Here's how the part is built. I have some questions about the finished solid (model axes, mm). Coordinates: 2 decimals unless noted, no trailing zeros. Write each loop counter-clockwise with the first axis right and the second up, starting at its lowest first coordinate (ties: lowest second). Pieces come first, ordered by that corner, then holes. Notation, with made-up numbers: (30.5, 76) -> (35.5, 76) arc R25 ccw to (35.5, 99) -> close; hole circle Ø6 at (37.25, 5.25). An arc over 180 degrees is marked (long way). Answer in a Markdown table with one row per item. Add a question column.
from build123d import *

# Parameters (mm, degrees)
BOSS_EXTRUDE1_DEPTH = 133.35
SKETCH2_R           = 21
CUT_EXTRUDE1_DEPTH  = 187.593999065
SKETCH3_W           = 133.35
SKETCH3_H           = 3.175
BOSS_EXTRUDE2_DEPTH = 3.175
FILLET1_R           = 3.175
SKETCH5_R           = 15
CUT_EXTRUDE2_DEPTH  = 189.467318942
SKETCH6_R           = 6.0325
CUT_EXTRUDE3_DEPTH  = 189.467318942
SKETCH7_R           = 3.175
CUT_EXTRUDE4_DEPTH  = 189.472240296
SKETCH15_R          = 2.5
CUT_EXTRUDE8_DEPTH  = 189.467318942
SKETCH18_R          = 30.1625
SKETCH18_R_2        = 21
BOSS_EXTRUDE3_DEPTH = 2.688354466


with BuildPart() as part:
    # Sketch1 → Boss-Extrude1 (new body)
    with BuildSketch(Plane.XY):
        Polygon((110.49, -69.425000088), (0, 0), (0, 3.175), (110.49, -66.250000088), align=None)
    extrude(amount=BOSS_EXTRUDE1_DEPTH)

    # Sketch2 → Cut-Extrude1 (cut, through all)
    with BuildSketch(Plane(origin=(1.430283892, 2.276299128, 0), x_dir=(0.8467258159330607, -0.5320295035357462, 0), z_dir=(0.5320295035357462, 0.8467258159330607, 0))):
        with Locations(Location((42.760806326, -41.91, 0), (0, 0, 180))):
            Circle(SKETCH2_R)
    extrude(amount=-CUT_EXTRUDE1_DEPTH, mode=Mode.SUBTRACT)

    # Sketch3 → Boss-Extrude2 (add)
    with BuildSketch(Plane(origin=(110.49, 0, 0), x_dir=(0, 0, -1), z_dir=(1, 0, 0))):
        with Locations((-66.675, -67.837500088)):
            Rectangle(SKETCH3_W, SKETCH3_H)
    extrude(amount=BOSS_EXTRUDE2_DEPTH)

    # Fillet1
    fillet1_edges = [part.edges().sort_by_distance(p)[0] for p in [
        (113.665, -66.250000088, 66.675),
    ]]
    fillet(fillet1_edges, radius=FILLET1_R - 0.0001)  # a hair under: the kernel refuses the full size

    # Sketch5 → Cut-Extrude2 (cut, through all)
    with BuildSketch(Plane(origin=(1.430283892, 2.276299128, 0), x_dir=(0.8467258159330606, -0.5320295035357464, 0), z_dir=(0.5320295035357464, 0.8467258159330606, 0))):
        with Locations(Location((17.360806326, -101.6, 0), (0, 0, 180))):
            Circle(SKETCH5_R)
        with Locations(Location((58.000806326, -101.6, 0), (0, 0, 180))):
            Circle(SKETCH5_R)
    extrude(amount=-CUT_EXTRUDE2_DEPTH, mode=Mode.SUBTRACT)

    # Sketch6 → Cut-Extrude3 (cut, through all)
    with BuildSketch(Plane(origin=(1.430283892, 2.276299128, 0), x_dir=(0.8467258159330606, -0.5320295035357464, 0), z_dir=(0.5320295035357464, 0.8467258159330606, 0))):
        with Locations(Location((90.701690059, -66.675, 0), (0, 0, 180))):
            Circle(SKETCH6_R)
        with Locations(Location((90.701690059, -47.625, 0), (0, 0, 180))):
            Circle(SKETCH6_R)
        with Locations(Location((90.701690059, -28.575, 0), (0, 0, 180))):
            Circle(SKETCH6_R)
        with Locations(Location((90.701690059, -85.725, 0), (0, 0, 180))):
            Circle(SKETCH6_R)
        with Locations(Location((90.701690059, -104.775, 0), (0, 0, 180))):
            Circle(SKETCH6_R)
    extrude(amount=-CUT_EXTRUDE3_DEPTH, mode=Mode.SUBTRACT)

    # Sketch7 → Cut-Extrude4 (cut, through all)
    with BuildSketch(Plane(origin=(0, 0, 0), x_dir=(0.8467258159330607, -0.5320295035357464, 0), z_dir=(-0.5320295035357463, -0.8467258159330606, 0))):
        with Locations((105.090883732, 123.825)):
            Circle(SKETCH7_R)
        with Locations((25.4, 123.825)):
            Circle(SKETCH7_R)
        with Locations((25.4, 9.525)):
            Circle(SKETCH7_R)
        with Locations((105.090883732, 9.525)):
            Circle(SKETCH7_R)
    extrude(amount=-CUT_EXTRUDE4_DEPTH, mode=Mode.SUBTRACT)

    # Sketch15 → Cut-Extrude8 (cut, through all)
    with BuildSketch(Plane(origin=(1.430283892, 2.276299128, 0), x_dir=(0.8467258159330606, -0.5320295035357464, 0), z_dir=(0.5320295035357464, 0.8467258159330606, 0))):
        with Locations(Location((17.360806326, -76.2, 0), (0, 0, 180))):
            Circle(SKETCH15_R)
        with Locations(Location((76.731690059, -66.675, 0), (0, 0, 180))):
            Circle(SKETCH15_R)
        with Locations(Location((58.000806326, -76.2, 0), (0, 0, 180))):
            Circle(SKETCH15_R)
    extrude(amount=-CUT_EXTRUDE8_DEPTH, mode=Mode.SUBTRACT)

    # Sketch18 → Boss-Extrude3 (add)
    with BuildSketch(Plane(origin=(1.430283892, 2.276299128, 0), x_dir=(0.8467258159330606, -0.5320295035357464, 0), z_dir=(0.5320295035357464, 0.8467258159330606, 0))):
        with Locations((42.760806326, -41.91)):
            Circle(SKETCH18_R)
        with Locations(Location((42.760806326, -41.91, 0), (0, 0, 180))):
            Circle(SKETCH18_R_2, mode=Mode.SUBTRACT)
    extrude(amount=-BOSS_EXTRUDE3_DEPTH)


solid = part.part
Q1. I need wall thicknesses on line 1 (Y direction, x = 48.5, z = 85); line 2 (Y direction, x = 29, z = 102); line 3 (X direction, y = -33, z = 59). Which ranges of each line are inside material? Lowest first, please. Write a range as [from, to].
Q2. Imagine slicing it at B-B on x = 50.5. State how many separate pieces and enclosed holes the cut face has, plus the area to 3 significant figures.
Q3. If we mould it in two halves opening along X, with no side actions, what happens to faces 1 (the flat face through (52, -31, 0)), 2 (the flat face through (54.47, -31.05, 65.74)), 3 (the cylindrical face through (89.106, -54.423, 120.726))? For each: pulls with the +X half, pulls with the -X half, needs draft (parallel to the pull), parting line crosses it, or undercut.
Q4. Imagine slicing it at D-D on y = -63. Please give me the cut outline in (x, z).
Q5. I'm going to push flat-ended pins straight in: P1, Ø6, axis at x = 69, z = 40.5, coming from the -Y side; P2, Ø6, axis at y = -52, z = 46.5, coming from the -X side; P3, Ø2, axis at x = 40.5, z = 64, coming from the -Y side. Where does each tip first touch, or does it pass through?
Result sheet:
| question | item | result |
|---|---|---|
| 1 | line 1 | y = [-30.47, -27.3] |
| 1 | line 2 | y = [-18.22, -15.05] |
| 1 | line 3 | x = [52.52, 57.57] |
| 2 | separate pieces | 4 |
| 2 | enclosed holes | 0 |
| 2 | area | 228 mm^2 |
| 3 | face 1 | needs draft |
| 3 | face 2 | pulls with the +X half |
| 3 | face 3 | undercut |
| 4 | outline | (100.26, 0) -> (105.32, 0) -> (105.32, 133.35) -> (100.26, 133.35) -> close |
| 5 | P1 | stops at y = -45.24 |
| 5 | P2 | stops at x = 80.74 |
| 5 | P3 | stops at y = -26.08 |
